Autodesk Inventor part; units mm, degrees
ref_plane "YZ Plane" through (0, 0, 0) normal (1, 0, 0) x (0, 1, 0)
ref_plane "XZ Plane" through (0, 0, 0) normal (0, 1, 0) x (-1, 0, 0)
ref_plane "XY Plane" through (0, 0, 0) normal (0, 0, 1) x (1, 0, 0)
sketch "Sketch1" plane through (0, 0, 0) normal (0, 0, 1) x (1, 0, 0)
  line L0 (-50, -50) -> (0, 0)
  line L1 (125, 0) -> (0, 0)
  line L2 (125, 0) -> (175, -50)
  line L3 (178, -50) -> (175, -50)
  line L4 (-53, -50) -> (-50, -50)
  circle A0 centre (117.5, -37.5) radius 1.5
  arc A1 (114.25, -43.8002) -> (114.25, -56.1998) centre (117.5, -50) ccw
  arc A2 (120.75, -56.1998) -> (120.75, -43.8002) centre (117.5, -50) ccw
  line L5 (-53, -50) -> (0, 3)
  line L6 (0, 3) -> (125, 3)
  line L7 (125, 3) -> (178, -50)
extrude "Extrusion1" add sketch "Sketch1" along normal blind 44.125 contours L4 L5 L6 L7 L3 L2 L1 L0
sketch "Sketch2" plane through (0, 3, 0) normal (0, 1, 0) x (1, 0, 0)
  line L0 (0, 0) -> (125, 0)
  line L1 (125, -10) -> (0, -10)
  circle A0 centre (31.25, -5) radius 1.8
  circle A1 centre (93.75, -5) radius 1.8
  line L2 (-53, 32.375) -> (-53, -10)
  line L3 (-53, -10) -> (-50, -10)
  line L4 (-50, -10) -> (0, -10)
  line L5 (0, 0) -> (-53, 0)
  line L6 (-53, 0) -> (-53, -44.125)
  line L7 (0, -44.125) -> (-53, -44.125)
  line L8 (0, 0) -> (0, -44.125)
  circle A2 centre (31.25, -5) radius 1.6
  circle A3 centre (93.75, -5) radius 1.6
  line L9 (125, 0) -> (0, 0)
  line L10 (0, 0) -> (0, -44.125)
  line L11 (125, -44.125) -> (0, -44.125)
  line L12 (125, 0) -> (125, -44.125)
  dimension "d2" = 3.2
  dimension "d3" = 3.2
extrude "Extrusion2" cut sketch "Sketch2" against normal up to surface (3 mm away) contours A0 | A1 | A2 | A3
chamfer "Chamfer2" distance 10 angle 45 1 edges at (-51.5, -50, 44.125)
properties part number "obudowa_górna_dluga" material "ABS Plastic"
Geometry check sheet. Reference: the model listing, model coordinates, mm. A direction names the side the tool comes from. Give positions to 0.01 mm unless a question says otherwise; leave off trailing zeros. Loops run counter-clockwise (first coordinate to the right, second up) from the corner with the lowest first, then second, coordinate; pieces in that order, holes last. Notation, with made-up numbers: M -15.5,86 L -5.5,86 A18 cw -5.5,101 Z; hole C -27.5,-12.75 d6. An arc over 180 degrees is marked long. Answer as CSV lines item,"result".
Item 1: Material ranges on line 1 (Z direction, x = 31.25, y = 1.65) (3 decimals); line 2 (X direction, y = 2, z = 5); line 3 (X direction, y = 1.1, z = 5), recorded low to high.
Values:
line 1,"z = 0 to 3.2, 6.8 to 44.125"
line 2,"x = -1 to 29.45, 33.05 to 91.95, 95.55 to 126"
line 3,"x = -1.9 to 29.45, 33.05 to 91.95, 95.55 to 126.9"
Item 2: Cross-section at B-B on z = 18. Record the cut outline in (x, y), and give its area (3 significant figures).
Values:
outline,"M -53,-50 L -50,-50 L 0,0 L 125,0 L 175,-50 L 178,-50 L 125,3 L 0,3 Z"
area,"684 mm²"
Item 3: Depth check by flat-ended pin: P1, Ø10, axis at y = -2.5, z = 20.5, coming from the -X side; P2, Ø6, axis at x = 51.5, z = 19.5, coming from the -Y side; P3, Ø4, axis at y = -41, z = 20.5, coming from the -X side; P4, Ø4.5, axis at x = 31.25, z = 5, coming from the +Y side. Enter the tip coordinate at first touch or a pass-through.
Values:
P1,"stops at x = -10.5"
P2,"stops at y = 0"
P3,"stops at x = -46"
P4,"stops at y = 3"
Item 4: Release check for a two-part mould opening along X. For faces 4 (the flat face through (150, -25, 22)), 5 (the flat face through (151, -23, 22)), 6 (the flat face through (63, 0, 22)), 7 (the flat face through (-27, -24, 22)) record: pulls with the +X half, pulls with the -X half, needs draft (parallel to the pull), parting line crosses it, or undercut.
Values:
face 4,"undercut"
face 5,"pulls with the +X half"
face 6,"undercut"
face 7,"pulls with the -X half"
Item 5: Cross-section at C-C on x = 104. Record the cut outline in (y, z) (3 decimals), and give its area (3 significant figures).
Values:
outline,"M 0,0 L 3,0 L 3,44.125 L 0,44.125 Z"
area,"132 mm²"
Item 6: Cross-section at A-A on y = -23. Record the cut outline in (x, z) (3 decimals), and give its area (3 significant figures).
Values:
outline,"M -26,0 L -23,0 L -23,44.125 L -26,44.125 Z; M 148,0 L 151,0 L 151,44.125 L 148,44.125 Z"
area,"265 mm²"
Item 7: Cross-section at D-D on z = 38.5. Record the cut outline in (x, y) (3 decimals), and give its area (3 significant figures).
Values:
outline,"M -48.625,-45.625 L -45.625,-45.625 L 0,0 L 125,0 L 175,-50 L 178,-50 L 125,3 L 0,3 Z"
area,"671 mm²"
Item 8: Access from +Z, -Z, +X, -X, +Y, -Y to the whole of each face (thin tool, end or side, straight path). Record for faces 1 (the flat face through (-46.53, -45.023, 39.102)), 2 (the flat face through (-25, -25, 22)), 3 (the flat face through (62, 3, 22)).
Values:
face 1,"+Z, -X, -Y"
face 2,"+Z, -Z, -Y"
face 3,"+Z, -Z, +X, -X, +Y"
